Source: CAD feature listing. Evaluate the final solid. Frame: model axes, mm. A direction names the side the tool comes from. Round coordinates to 2 decimals unless told otherwise and drop trailing zeros. Write each loop counter-clockwise with the first axis right and the second up, starting at its lowest first coordinate (ties: lowest second). Pieces come first, ordered by that corner, then holes. Notation, with made-up numbers: M 36,89.5 L 92,89.5 A18 cw 92,102.5 Z; hole C -24.75,-16 d8. An arc over 180 degrees is marked long. Use a Markdown table: item, result.
```python
from build123d import *

# Parameters (mm, degrees)
SKETCH1_W           = 144.5
SKETCH1_H           = 172.38
BOSS_EXTRUDE1_DEPTH = 38
SKETCH2_R           = 10.5
SKETCH2_R_2         = 1.99
CUT_EXTRUDE1_DEPTH  = 39
CUT_EXTRUDE2_DEPTH  = 2
SKETCH4_R           = 15.25
CUT_EXTRUDE3_DEPTH  = 20


with BuildPart() as part:
    # Sketch1 → Boss-Extrude1 (new body)
    with BuildSketch(Plane(origin=(0, 0, 0), x_dir=(1, 0, 0), z_dir=(0, 1, 0))):
        Rectangle(SKETCH1_W, SKETCH1_H)
    extrude(amount=BOSS_EXTRUDE1_DEPTH)

    # Sketch2 → Cut-Extrude1 (cut, through all)
    with BuildSketch(Plane.XZ):
        with Locations((-42.25, -56.19)):
            Circle(SKETCH2_R)
        with Locations((10.25, -56.19)):
            Circle(SKETCH2_R_2)
        with Locations((42.25, -56.19)):
            Circle(SKETCH2_R)
        with Locations((-42.25, 56.19)):
            Circle(SKETCH2_R)
        with Locations((-10.25, 56.19)):
            Circle(SKETCH2_R_2)
        with Locations((42.25, 56.19)):
            Circle(SKETCH2_R)
        Polygon((57.25, -20.94), (67.25, -20.94), (67.25, -17.44), (65.25, -17.44), (65.25, -17.94), (59.25, -17.94), (59.25, -17.44), (57.25, -17.44), align=None)
        with BuildLine():
            Line((-1.333860018, -0.707106781), (-10.455537495, -9.828784258))
            ThreePointArc((-10.455537495, -9.828784258), (-10.455537495, -13.647160877), (-6.637160877, -13.647160877))
            Line((-6.637160877, -13.647160877), (7.01, 0))
            Line((7.01, 0), (-6.637160877, 13.647160877))
            ThreePointArc((-6.637160877, 13.647160877), (-10.455537495, 13.647160877), (-10.455537495, 9.828784258))
            Line((-10.455537495, 9.828784258), (-1.333860018, 0.707106781))
            ThreePointArc((-1.333860018, 0.707106781), (0.373246763, 0), (-1.333860018, -0.707106781))
        make_face()
    extrude(amount=-CUT_EXTRUDE1_DEPTH, mode=Mode.SUBTRACT)

    # Sketch3 → Cut-Extrude2 (cut)
    with BuildSketch(Plane.XZ):
        Polygon((72.25, 17.44), (-72.25, 17.44), (-72.25, -17.94), (57.25, -17.94), (57.25, -17.44), (59.25, -17.44), (59.25, -17.94), (65.25, -17.94), (65.25, -17.44), (67.25, -17.44), (67.25, -20.94), (72.25, -20.94), align=None)
        with BuildLine():
            Line((7.01, 0), (-6.637160877, -13.647160877))
            ThreePointArc((-6.637160877, -13.647160877), (-10.455537495, -13.647160877), (-10.455537495, -9.828784258))
            Line((-10.455537495, -9.828784258), (-1.333860018, -0.707106781))
            ThreePointArc((-1.333860018, -0.707106781), (0.373246763, 0), (-1.333860018, 0.707106781))
            Line((-1.333860018, 0.707106781), (-10.455537495, 9.828784258))
            ThreePointArc((-10.455537495, 9.828784258), (-10.455537495, 13.647160877), (-6.637160877, 13.647160877))
            Line((-6.637160877, 13.647160877), (7.01, 0))
        make_face(mode=Mode.SUBTRACT)
    extrude(amount=-CUT_EXTRUDE2_DEPTH, mode=Mode.SUBTRACT)

    # Sketch4 → Cut-Extrude3 (cut)
    with BuildSketch(Plane(origin=(0, 38, 0), x_dir=(1, 0, 0), z_dir=(0, 1, 0))):
        with Locations((-42.25, 56.19)):
            Circle(SKETCH4_R)
        with Locations((42.25, 56.19)):
            Circle(SKETCH4_R)
        with Locations((42.25, -56.19)):
            Circle(SKETCH4_R)
        with Locations((-42.25, -56.19)):
            Circle(SKETCH4_R)
    extrude(amount=-CUT_EXTRUDE3_DEPTH, mode=Mode.SUBTRACT)


solid = part.part
```
Q1. Section C-C on y = 24.5. Give the number of separate pieces and of enclosed holes in the cut face, plus the area to 3 significant figures.
Results are:
| item | result |
|---|---|
| separate pieces | 1 |
| enclosed holes | 8 |
| area | 21,700 mm^2 |
Q2. Section B-B on x = -42.25. Return loops of the section in (y, z), plus the area to 3 significant figures.
Results are:
| item | result |
|---|---|
| outline | M 0,-86.19 L 38,-86.19 L 38,-71.44 L 18,-71.44 L 18,-66.69 L 0,-66.69 Z; M 0,-45.69 L 18,-45.69 L 18,-40.94 L 38,-40.94 L 38,40.94 L 18,40.94 L 18,45.69 L 0,45.69 L 0,17.44 L 2,17.44 L 2,-17.94 L 0,-17.94 Z; M 0,66.69 L 18,66.69 L 18,71.44 L 38,71.44 L 38,86.19 L 0,86.19 Z |
| area | 4,500 mm^2 |
Q3. First-contact query: pin 1 Ø19 at (x, z) = (9.5, 7) entering from -Y; pin 2 Ø15 at (x, z) = (-41, -53) entering from +Y. Flat tips, straight axial feed; report the tip coordinate or a pass-through.
Results are:
| item | result |
|---|---|
| pin 1 | y = 2 |
| pin 2 | y = 18 |
Q4. Reachability of faces 5 (the cylindrical face through (31.01, 28.14, -66.497)), 6 (the flat face through (-17, 38, -1)), 7 (the flat face through (67.25, 20, -19)) from +Z, -Z, +X, -X, +Y, -Y: full face, straight path, thin tool, end or side. Return the list, or none.
Results are:
| item | result |
|---|---|
| face 5 | +Y |
| face 6 | +Z, -Z, +X, -X, +Y |
| face 7 | +Y, -Y |
Q5. Mould query, pull axis X, two halves, no side actions, for faces 1 (the flat face through (-72.25, 19, 1)), 2 (the flat face through (-1, 0, -53)), 3 (the cylindrical face through (33.92, 8.87, -62.58)), 4 (the cylindrical face through (-50.58, 8.87, 49.8)). Classes: +X half, -X half, draft (parallel to the pull), parting line (faces both ways), or undercut.
Results are:
| item | result |
|---|---|
| face 1 | -X half |
| face 2 | draft |
| face 3 | undercut |
| face 4 | undercut |
Q6. Section A-A on z = -56.19. Return loops of the section in (x, y).
Results are:
| item | result |
|---|---|
| outline | M -72.25,0 L -52.75,0 L -52.75,18 L -57.5,18 L -57.5,38 L -72.25,38 Z; M -31.75,0 L 8.26,0 L 8.26,38 L -27,38 L -27,18 L -31.75,18 Z; M 12.24,0 L 31.75,0 L 31.75,18 L 27,18 L 27,38 L 12.24,38 Z; M 52.75,0 L 72.25,0 L 72.25,38 L 57.5,38 L 57.5,18 L 52.75,18 Z |
Q7. Section D-D on z = 5. Return loops of the section in (x, y), plus the area to 3 significant figures.
Results are:
| item | result |
|---|---|
| outline | M -72.25,2 L -5.63,2 L -5.63,38 L -72.25,38 Z; M 2.01,2 L 72.25,2 L 72.25,38 L 2.01,38 Z |
| area | 4,930 mm^2 |
Q8. Line query: L1, parallel to X at y = 32, z = 56; L2, parallel to X at y = 10, z = -56; L3, parallel to Z at x = 42, y = 7. Output: solid intervals per line, ascending.
Results are:
| item | result |
|---|---|
| L1 | -72.25 to -57.5, -27 to -12.23, -8.27 to 27, 57.5 to 72.25 |
| L2 | -72.25 to -52.75, -31.75 to 8.27, 12.23 to 31.75, 52.75 to 72.25 |
| L3 | -86.19 to -66.69, -45.69 to 45.69, 66.69 to 86.19 |
